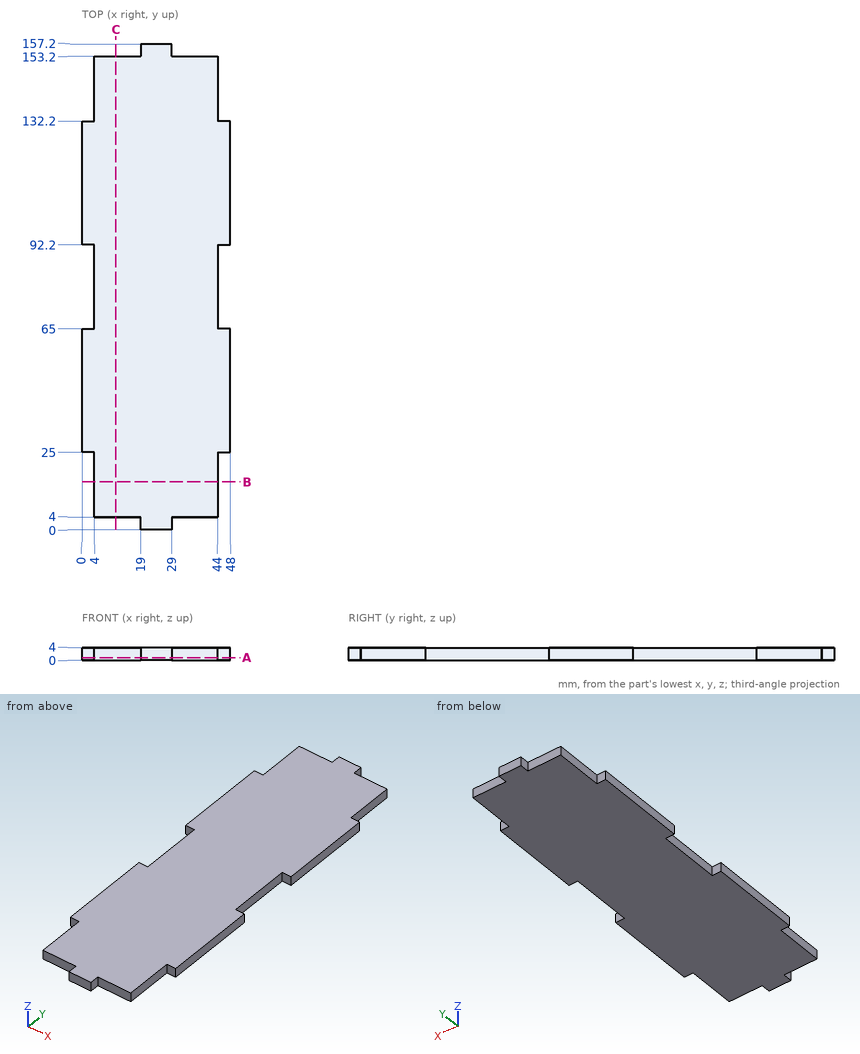
Source: three-view drawing plus pictorial views. Frame: mm from the lowest corner of the part. Give positions to 0.01 mm unless a question says otherwise; leave off trailing zeros. Order: outer loops, then holes, each group sorted by start corner. A loop starts at its lowest first (then second) coordinate and runs counter-clockwise, first axis right, second up.
1. Material intervals for L1, parallel to Y at x = 3, z = 0.9; L2, parallel to Y at x = 41, z = 1.85; L3, parallel to X at y = 148, z = 3.5, sorted ascending.
Derived:
L1: y = 25 to 65, 92.2 to 132.2
L2: y = 4 to 153.2
L3: x = 4 to 44
2. Pin query (flat end, axial travel): pin 1 (1.2 mm diameter, centred on x = 1, z = 1, fed in from -Y); pin 2 (2 mm diameter, centred on y = 142, z = 1.5, fed in from +X); pin 3 (1.2 mm diameter, centred on x = 9, z = 2, fed in from -Y). Return the tip coordinate at first contact, or that it passes through.
Derived:
pin 1: stops at y = 25
pin 2: stops at x = 44
pin 3: stops at y = 4
3. Section C-C on x = 11. Return the cut outline in (y, z).
Derived:
outline: (4, 0) - (153.2, 0) - (153.2, 4) - (4, 4) - close
4. Section A-A on z = 0.8. Return the cut outline in (x, y).
Derived:
outline: (0, 25) - (4, 25) - (4, 4) - (19, 4) - (19, 0) - (29, 0) - (29, 4) - (44, 4) - (44, 25) - (48, 25) - (48, 65) - (44, 65) - (44, 92.2) - (48, 92.2) - (48, 132.2) - (44, 132.2) - (44, 153.2) - (29, 153.2) - (29, 157.2) - (19, 157.2) - (19, 153.2) - (4, 153.2) - (4, 132.2) - (0, 132.2) - (0, 92.2) - (4, 92.2) - (4, 65) - (0, 65) - close
5. Section B-B on y = 15.5. Return the cut outline in (x, z), and give its area (3 significant figures).
Derived:
outline: (4, 0) - (44, 0) - (44, 4) - (4, 4) - close
area: 160 mm2
